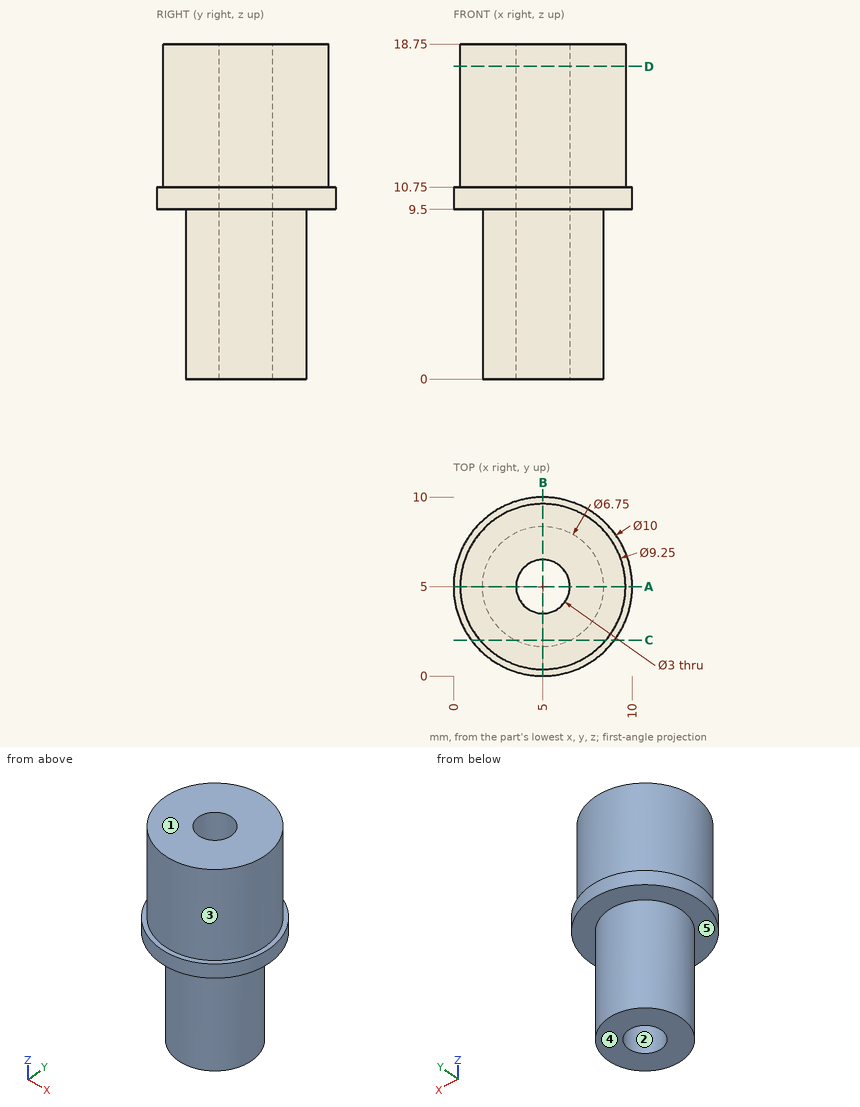
Job drawing, mm, ordinate dimensions from the low corner. One solid piece. A direction names the side the tool comes from. Coordinates: 2 decimals unless noted, no trailing zeros. Write each loop counter-clockwise with the first axis right and the second up, starting at its lowest first coordinate (ties: lowest second). Pieces come first, ordered by that corner, then holes.
Item 1: Pin check, flat tips, straight feed: pin 1 (1 mm diameter, centred on x = 7.5, z = 7.5, fed in from -Y); pin 2 (2 mm diameter, centred on y = 3, z = 2.5, fed in from -X). Stop position of each tip, or through.
Item 2: Mould opens along X. For the marked faces 1, 2 and 3 say: released by +X, released by -X, zero draft, split by the parting line, or undercut.
Item 3: Probe line 1 (Y direction, x = 5, z = 7.75) (3 decimals); line 2 (Y direction, x = 5, z = 15) (3 decimals); line 3 (Z direction, x = 2.25, y = 2.75). List the from-to ranges inside material, lowest first.
Item 4: Which spindle directions (+Z, -Z, +X, -X, +Y, -Y) get a long thin tool onto all of the face, cutting with end or side? Do the marked faces 4 and 5. Say none if no direction does.
Item 5: Slice it at C-C (y = 2). Write the cut outline in (x, z), and give its area (3 significant figures).
Item 6: Slice it at A-A (y = 5). Write the cut outline in (x, z) (3 decimals), and give its area (3 significant figures).
Item 7: Slice it at D-D (z = 17.5). Write the cut outline in (x, y) (3 decimals), and give its area (3 significant figures).
Results found:
1. pin 1: stops at y = 2.28
1. pin 2: stops at x = 1.78
2. face 1: zero draft
2. face 2: undercut
2. face 3: split by the parting line
3. line 1: y = 1.625 to 3.5, 6.5 to 8.375
3. line 2: y = 0.375 to 3.5, 6.5 to 9.625
3. line 3: z = 9.5 to 18.75
4. face 4: -Z, +X, -X, +Y, -Y
4. face 5: -Z
5. outline: (1, 9.5) - (3.45, 9.5) - (3.45, 0) - (6.55, 0) - (6.55, 9.5) - (9, 9.5) - (9, 10.75) - (8.52, 10.75) - (8.52, 18.75) - (1.48, 18.75) - (1.48, 10.75) - (1, 10.75) - close
5. area: 95.7 mm2
6. outline: (0, 9.5) - (1.625, 9.5) - (1.625, 0) - (3.5, 0) - (3.5, 18.75) - (0.375, 18.75) - (0.375, 10.75) - (0, 10.75) - close; (6.5, 0) - (8.375, 0) - (8.375, 9.5) - (10, 9.5) - (10, 10.75) - (9.625, 10.75) - (9.625, 18.75) - (6.5, 18.75) - close
6. area: 94.4 mm2
7. outline: circle Ø9.25 at (5, 5); hole circle Ø3 at (5, 5)
7. area: 60.1 mm2
